```python
from build123d import *

# Parameters (mm, degrees)
F3_DEPTH = 45.001
F5_D     = 14
F6_R     = 2
F7_R     = 1
F8_SIZE  = 1
F9_R     = 0.5
F10_R    = 0.4


with BuildPart() as f1:
    # F0 (on Right) → F1 (revolve)
    with BuildSketch(Plane.YZ):
        Polygon((-2, 26), (0, 26), (0, 62.5), (-18, 62.5), (-18, 28), (-45, 28), (-45, 16), (-2, 16), align=None)
    revolve(axis=Axis((0, -22.398166, 0), (0, 1, 0)))

    # F2 (on face) → F3 (cut, through all)
    with BuildSketch(Plane.XZ.offset(45)):
        with BuildLine():
            ThreePointArc((4, 15.491933), (0, 16), (-4, 15.491933))
            Line((-4, 15.491933), (-4, 12))
            Line((-4, 12), (4, 12))
            Line((4, 12), (4, 15.491933))
        make_face()
        with BuildLine():
            Line((4, 18.4), (-4, 18.4))
            Line((-4, 18.4), (-4, 15.491933))
            ThreePointArc((-4, 15.491933), (0, 16), (4, 15.491933))
            Line((4, 15.491933), (4, 18.4))
        make_face()
    extrude(amount=-F3_DEPTH, mode=Mode.SUBTRACT)

    # F5 (through all)
    with Locations(Plane.XZ.offset(18)):
        with Locations((30.052038, 30.052038), (30.052038, -30.052038), (-30.052038, -30.052038), (-30.052038, 30.052038)):
            Hole(F5_D / 2)

    # F6
    f6_edges = [f1.edges().sort_by_distance(p)[0] for p in [
        (0, -18, -28),
        (0, -45, -28),
    ]]
    fillet(f6_edges, radius=F6_R)

    # F7
    f7_edges = [f1.edges().sort_by_distance(p)[0] for p in [
        (0, -18, -62.5),
    ]]
    fillet(f7_edges, radius=F7_R)

    # F8
    f8_edges = [f1.edges().sort_by_distance(p)[0] for p in [
        (0, 0, -62.5),
    ]]
    chamfer(f8_edges, length=F8_SIZE)

    # F9
    f9_edges = [f1.edges().sort_by_distance(p)[0] for p in [
        (0, 0, -26),
    ]]
    fillet(f9_edges, radius=F9_R)

    # F10
    f10_edges = [f1.edges().sort_by_distance(p)[0] for p in [
        (0, -2, -26),
    ]]
    fillet(f10_edges, radius=F10_R)


solid = f1.part
```
The listing builds one solid part. Answer for the finished solid, in the listing's coordinates (mm). A direction names the side the tool comes from. Coordinates: 2 decimals unless noted, no trailing zeros. Write each loop counter-clockwise with the first axis right and the second up, starting at its lowest first coordinate (ties: lowest second). Pieces come first, ordered by that corner, then holes. Notation, with made-up numbers: (89.5, 53.5) - (119.5, 53.5) arc R6 ccw to (119.5, 58.5) - close; hole circle Ø1 at (49.25, 69.5). An arc over 180 degrees is marked (long way). Return JSON: item names as keys, results as strings. Group by question number.
1. A cutting plane is placed at C-C, the plane y = -41. Determine the outline of the cut face in (x, z), plus the area to 3 significant figures.
2. A cutting plane is placed at A-A, the plane x = 0. Determine the outline of the cut face in (y, z).
3. Given pin 1 (8 mm diameter, centred on x = -45.5, z = -43, fed in from +Y); pin 2 (4 mm diameter, centred on x = 0, y = -34, fed in from -Z); pin 3 (1 mm diameter, centred on x = -8.5, z = -33.5, fed in from -Y); pin 4 (2 mm diameter, centred on y = -17, z = -0.5, fed in from +X), each flat-ended and moving along its own axis, determine where each tip first touches the part or whether it passes through.
4. Straight lines are drawn through the part: L1, parallel to X at y = -3, z = 35.5; L2, parallel to X at y = -24, z = 0; L3, parallel to X at y = -2.5, z = 31.5. For each, find the intervals that lie inside material, in ascending order.
5. Which of the six approach directions +Z, -Z, +X, -X, +Y, -Y give full straight-line access (tool end or side, diameter ignored) to faces 1 (the flat face through (12, -2, -11)), 2 (the flat face through (-11, -45, -12)), 3 (the flat face through (0, -24, 18.4))?
6. A cutting plane is placed at D-D, the plane y = -12. Determine the outline of the cut face in (x, z).
7. Determine the mould class of faces 4 (the flat face through (4, -24, 17)), 5 (the cylindrical face through (-10.724, -31.661, 25.865)), 6 (the flat face through (14.5, -18, 26.5)) for opening direction Z: released by +Z, released by -Z, zero draft, split by the parting line, or undercut.
8. A cutting plane is placed at B-B, the plane z = 0. Determine the outline of the cut face in (x, y), plus the area to 3 significant figures.
Ans:
{
 "1": {"outline": "circle Ø56 at (0, 0); hole (-4, 15.49) arc R16 ccw (long way) to (4, 15.49) - (4, 18.4) - (-4, 18.4) - close", "area": "1,640 mm²"},
 "2": {"outline": "(-45, -26) arc R2 ccw to (-43, -28) - (-20, -28) arc R2 cw to (-18, -30) - (-18, -61.5) arc R1 ccw to (-17, -62.5) - (-1, -62.5) - (0, -61.5) - (0, -26.5) arc R0.5 ccw to (-0.5, -26) - (-1.6, -26) arc R0.4 cw to (-2, -25.6) - (-2, -16) - (-45, -16) - close; (-45, 18.4) - (-2, 18.4) - (-2, 25.6) arc R0.4 cw to (-1.6, 26) - (-0.5, 26) arc R0.5 ccw to (0, 26.5) - (0, 61.5) - (-1, 62.5) - (-17, 62.5) arc R1 ccw to (-18, 61.5) - (-18, 30) arc R2 cw to (-20, 28) - (-43, 28) arc R2 ccw to (-45, 26) - close"},
 "3": {"pin 1": "y = 0", "pin 2": "z = -28", "pin 3": "y = -18", "pin 4": "x = 62.5"},
 "4": {"L1": "-51.44 to -34.45, -25.66 to 25.66, 34.45 to 51.44", "L2": "-28 to -16, 16 to 28", "L3": "-53.98 to -36.9, -23.2 to 23.2, 36.9 to 53.98"},
 "5": {"face 1": "+Y", "face 2": "+Z, -Z, +X, -X, -Y", "face 3": "+Y, -Y"},
 "6": {"outline": "circle Ø125 at (0, 0); hole circle Ø14 at (-30.05, -30.05); hole circle Ø14 at (-30.05, 30.05); hole (-4, 15.49) arc R16 ccw (long way) to (4, 15.49) - (4, 18.4) - (-4, 18.4) - close; hole circle Ø14 at (30.05, -30.05); hole circle Ø14 at (30.05, 30.05)"},
 "7": {"face 4": "undercut", "face 5": "split by the parting line", "face 6": "zero draft"},
 "8": {"outline": "(-62.5, -17) arc R1 ccw to (-61.5, -18) - (-30, -18) arc R2 cw to (-28, -20) - (-28, -43) arc R2 ccw to (-26, -45) - (-16, -45) - (-16, -2) - (-25.6, -2) arc R0.4 cw to (-26, -1.6) - (-26, -0.5) arc R0.5 ccw to (-26.5, 0) - (-61.5, 0) - (-62.5, -1) - close; (16, -45) - (26, -45) arc R2 ccw to (28, -43) - (28, -20) arc R2 cw to (30, -18) - (61.5, -18) arc R1 ccw to (62.5, -17) - (62.5, -1) - (61.5, 0) - (26.5, 0) arc R0.5 ccw to (26, -0.5) - (26, -1.6) arc R0.4 cw to (25.6, -2) - (16, -2) - close", "area": "2,280 mm²"}
}
